Solid Edge part; units mm, degrees
sketch "Sketch1" plane through (0, 0, 0) normal (0, -1, 0) x (1, 0, 0)
  arc A0 (-4.6736, 4.1) -> (5.8626, 5.0354) centre (1, 0) cw
  line L0 (5.8626, 5.0354) -> (8.9488, 2.0551)
  line L1 (5.8626, -5.0354) -> (8.9488, -2.0551)
  arc A1 (5.8626, -5.0354) -> (-4.6736, -4.1) centre (1, 0) cw
  line L2 (1, -4.1) -> (-4.6736, -4.1)
  line L3 (1, 4.1) -> (-4.6736, 4.1)
  arc A2 (8.9488, -2.0551) -> (8.9488, 2.0551) centre (10.7, 0) cw
  arc A3 (1, 4.1) -> (1, -4.1) centre (1, 0) cw
extrude "Protrusion1" add sketch "Sketch1" along normal blind 6
extrude "ExtrudedCutout_1" [suppressed]
chamfer "Chamfer_1" distance 0.5 angle 45 8 edges at (5.1, -6, 0) (-1.8368, -6, 4.1) (-1.8368, -6, -4.1) (0.381, -6, 6.9726) (7.4057, -6, 3.5452) (7.4057, -6, -3.5452) (0.381, -6, -6.9726) (8, -6, 0)
properties material "ABS Plastic, medium impact"
Here's how the part is built. I have some questions about the finished solid (model axes, mm). Give positions to 0.01 mm unless a question says otherwise; leave off trailing zeros. Loops run counter-clockwise (first coordinate to the right, second up) from the corner with the lowest first, then second, coordinate; pieces in that order, holes last. Notation, with made-up numbers: (28, -4.75) -> (83, -4.75) arc R17 ccw to (83, 24.25) -> close; hole circle Ø10 at (81.25, 18.5). An arc over 180 degrees is marked (long way). Answer as a JSON object with one key per item and string values. Group by question number.
Item 1: Imagine slicing it at B-B on z = 0. Write out the boundary of the cut face in (x, y), then the cut area to 4 significant figures.
Item 2: I need wall thicknesses on L1, parallel to Z at x = 1, y = -2.75; L2, parallel to Z at x = -2, y = -3.75; L3, parallel to Z at x = 5.25, y = -2. Which ranges of each line are inside material? Lowest first, please.
Item 3: Thinking about a two-plate mould opening in Z: for faces 1 (the conical face through (5.24, -5.64, -0.09)), 2 (the conical face through (0.49, -5.86, -6.62)), 3 (the conical face through (0.333, -5.858, 6.609)), 4 (the conical face through (7.86, -5.64, 0.03)), which applies, pulls with the +Z half, pulls with the -Z half, needs draft (parallel to the pull), parting line crosses it, or undercut?
Item 4: Will these pins go through, and if not, where does the flat tip stop? pin 1 (3 mm diameter, centred on x = 0, y = -3, fed in from -Z); pin 2 (1 mm diameter, centred on x = 6, y = -4.5, fed in from +Z); pin 3 (3 mm diameter, centred on x = -1, y = -2, fed in from +Z); pin 4 (3 mm diameter, centred on x = -3, y = -2.5, fed in from -Z).
Item 5: Imagine slicing it at A-A on y = -0.25. Write out the boundary of the cut face in (x, z).
Answer list:
{
 "1": {"outline": "(5.1, -5.5) -> (5.6, -6) -> (7.5, -6) -> (8, -5.5) -> (8, 0) -> (5.1, 0) -> close", "area": "17.15 mm2"},
 "2": {"L1": "z = -7 to -4.1, 4.1 to 7", "L2": "z = -6.32 to -4.1, 4.1 to 6.32", "L3": "z = -5.56 to 5.56"},
 "3": {"face 1": "undercut", "face 2": "pulls with the -Z half", "face 3": "pulls with the +Z half", "face 4": "undercut"},
 "4": {"pin 1": "stops at z = -7", "pin 2": "stops at z = 5.36", "pin 3": "stops at z = 6.98", "pin 4": "stops at z = -6.54"},
 "5": {"outline": "(-4.67, -4.1) arc R7 ccw to (5.86, -5.04) -> (8.95, -2.06) arc R2.7 cw to (8.95, 2.06) -> (5.86, 5.04) arc R7 ccw to (-4.67, 4.1) -> (1, 4.1) arc R4.1 cw to (1, -4.1) -> close"}
}
